from build123d import *

# Parameters (mm, degrees)
BOSS_EXTRUDE1_DEPTH = 12


with BuildPart() as part:
    # Sketch1 → Boss-Extrude1 (new body)
    with BuildSketch(Plane.XY):
        with BuildLine():
            Line((36.538461538, -42.187912088), (27.803617527, -42.187912088))
            ThreePointArc((27.803617527, -42.187912088), (24.032111316, -41.72295633), (24.538461538, -45.489128447))
            Line((24.538461538, -45.489128447), (24.538461538, -78.187912088))
            Line((24.538461538, -78.187912088), (-3.461538462, -78.187912088))
            ThreePointArc((-3.461538462, -78.187912088), (-45.887945333, -60.614318959), (-63.461538462, -18.187912088))
            Line((-63.461538462, -18.187912088), (-63.461538462, 317.812087912))
            Line((-63.461538462, 317.812087912), (24.538461538, 317.812087912))
            Line((24.538461538, 317.812087912), (24.538461538, 285.113304271))
            ThreePointArc((24.538461538, 285.113304271), (24.032111316, 281.347132154), (27.803617527, 281.812087912))
            Line((27.803617527, 281.812087912), (36.538461538, 281.812087912))
            Line((36.538461538, 281.812087912), (36.538461538, 245.812087912))
            Line((36.538461538, 245.812087912), (27.803617527, 245.812087912))
            ThreePointArc((27.803617527, 245.812087912), (24.032111316, 246.27704367), (24.538461538, 242.510871553))
            Line((24.538461538, 242.510871553), (24.538461538, 213.113304271))
            ThreePointArc((24.538461538, 213.113304271), (24.032111316, 209.347132154), (27.803617527, 209.812087912))
            Line((27.803617527, 209.812087912), (36.538461538, 209.812087912))
            Line((36.538461538, 209.812087912), (36.538461538, 173.812087912))
            Line((36.538461538, 173.812087912), (27.803617527, 173.812087912))
            ThreePointArc((27.803617527, 173.812087912), (24.032111316, 174.27704367), (24.538461538, 170.510871553))
            Line((24.538461538, 170.510871553), (24.538461538, 164.212087912))
            Line((24.538461538, 164.212087912), (24.538461538, 141.113304271))
            ThreePointArc((24.538461538, 141.113304271), (24.032111316, 137.347132154), (27.803617527, 137.812087912))
            Line((27.803617527, 137.812087912), (36.538461538, 137.812087912))
            Line((36.538461538, 137.812087912), (36.538461538, 119.812087912))
            Line((36.538461538, 119.812087912), (36.538461538, 101.812087912))
            Line((36.538461538, 101.812087912), (27.803617527, 101.812087912))
            ThreePointArc((27.803617527, 101.812087912), (24.032111316, 102.27704367), (24.538461538, 98.510871553))
            Line((24.538461538, 98.510871553), (24.538461538, 75.412087912))
            Line((24.538461538, 75.412087912), (24.538461538, 69.113304271))
            ThreePointArc((24.538461538, 69.113304271), (24.032111316, 65.347132154), (27.803617527, 65.812087912))
            Line((27.803617527, 65.812087912), (36.538461538, 65.812087912))
            Line((36.538461538, 65.812087912), (36.538461538, 29.812087912))
            Line((36.538461538, 29.812087912), (27.803617527, 29.812087912))
            ThreePointArc((27.803617527, 29.812087912), (24.032111316, 30.27704367), (24.538461538, 26.510871553))
            Line((24.538461538, 26.510871553), (24.538461538, -2.886695729))
            ThreePointArc((24.538461538, -2.886695729), (24.032111316, -6.652867846), (27.803617527, -6.187912088))
            Line((27.803617527, -6.187912088), (36.538461538, -6.187912088))
            Line((36.538461538, -6.187912088), (36.538461538, -42.187912088))
        make_face()
    extrude(amount=BOSS_EXTRUDE1_DEPTH)


solid = part.part
The listing builds one solid part. Answer for the finished solid, in the listing's coordinates (mm). A direction names the side the tool comes from. Round coordinates to 2 decimals unless told otherwise and drop trailing zeros. Write each loop counter-clockwise with the first axis right and the second up, starting at its lowest first coordinate (ties: lowest second). Pieces come first, ordered by that corner, then holes. Notation, with made-up numbers: M 26.5,41.25 L 36.5,41.25 A27 ccw 36.5,64.25 Z; hole C -17.75,4.5 d10. An arc over 180 degrees is marked long. Write each question's results on one line, items separated by ' | '. Start each with the question number.
Item 1: Flat-ended cylindrical pins translate along their axes: pin 1 Ø4.5 at (x, y) = (25.74, 172.59) entering from -Z; pin 2 Ø4.5 at (x, z) = (34, 8.5) entering from +Y; pin 3 Ø3 at (x, z) = (-39.5, 8.5) entering from -Y; pin 4 Ø4.5 at (x, z) = (34, 8) entering from -Y. Find the tip coordinate at first contact, or state that the pin passes through.
Item 2: A cutting plane is placed at B-B on x = -40.5. Write down the section's boundary in (y, z).
Item 3: For a pull along Y with two mould halves and no side action, classify faces 4 (the face through (24.538, -62, 6)), 5 (the face through (24.538, 12, 6)), 6 (the face through (32, 281.812, 6)) as pulls with the +Y half, pulls with the -Y half, needs draft (parallel to the pull), parting line crosses it, or undercut.
Item 4: For faces 1 (the face through (-20, 317.812, 6)), 2 (the face through (32, 209.812, 6)), 3 (the face through (32, -42.188, 6)), determine the directions among +Z, -Z, +X, -X, +Y, -Y from which every point of the face is accessible in a straight line to the end or side of a thin tool.
Item 5: A cutting plane is placed at A-A on y = 217.5. Write down the section's boundary in (x, z), and give its area (3 significant figures).
Item 6: Straight lines are drawn through the part: L1, parallel to X at y = 244.5, z = 10.5; L2, parallel to X at y = -2.5, z = 3.25; L3, parallel to Y at x = -14, z = 3. For each, find the intervals that lie inside material, in ascending order. Write a range as [from, to].
Check sheet entries:
1) pin 1: through | pin 2: y = 281.81 | pin 3: y = -67.25 | pin 4: y = -42.19
2) outline: M -65.39,0 L 317.81,0 L 317.81,12 L -65.39,12 Z
3) face 4: needs draft | face 5: undercut | face 6: pulls with the +Y half
4) face 1: +Z, -Z, +X, -X, +Y | face 2: +Z, -Z, +X | face 3: +Z, -Z, +X, -Y
5) outline: M -63.46,0 L 24.54,0 L 24.54,12 L -63.46,12 Z | area: 1,060 mm²
6) L1: [-63.46, 23.34] | L2: [-63.46, 24.54] | L3: [-77.26, 317.81]
